Work out the finished part from the listing and answer in its coordinate system (mm). Give positions to 0.01 mm unless a question says otherwise; leave off trailing zeros. Order: outer loops, then holes, each group sorted by start corner. A loop starts at its lowest first (then second) coordinate and runs counter-clockwise, first axis right, second up. Notation, with made-up numbers: (82.25, 85) -> (104.25, 85) arc R12 cw to (104.25, 105) -> close; hole circle Ø6 at (-25.75, -5). An arc over 180 degrees is marked (long way). Use a Markdown table: item, result. Add a question column.
```python
from build123d import *

# Parameters (mm, degrees)
F0_R     = 2.25
F1_DEPTH = 15


with BuildPart() as f1:
    # F0 (on Top) → F1 (new body)
    with BuildSketch(Plane.XY):
        with BuildLine():
            ThreePointArc((20, 0), (18.535534, 3.535534), (15, 5))
            Line((15, 5), (-15, 5))
            ThreePointArc((-15, 5), (-18.535534, 3.535534), (-20, 0))
            ThreePointArc((-20, 0), (-18.535534, -3.535534), (-15, -5))
            Line((-15, -5), (15, -5))
            ThreePointArc((15, -5), (18.535534, -3.535534), (20, 0))
        make_face()
        with Locations((-15, 0)):
            Circle(F0_R, mode=Mode.SUBTRACT)
        with Locations((15, 0)):
            Circle(F0_R, mode=Mode.SUBTRACT)
    extrude(amount=F1_DEPTH)


solid = f1.part
```
1) The part is cut by section C-C, the plane y = 0.5. Determine the outline of the cut face in (x, z).
2) Determine the mould class of faces 1 (the flat face through (0, 0, 0)), 2 (the cylindrical face through (-12.854, 0.676, 7.395)) for opening direction X: released by +X, released by -X, zero draft, split by the parting line, or undercut.
3) The part is cut by section B-B, the plane z = 13.5. Determine the outline of the cut face in (x, y), then the cut area to 3 significant figures.
4) The part is cut by section A-A, the plane x = -16. Determine the outline of the cut face in (y, z), then the cut area to 3 significant figures.
5) Straight lines are drawn through the part: line 1 (Y direction, x = 15, z = 7.5); line 2 (X direction, y = -0.75, z = 5.5); line 3 (X direction, y = -2, z = 8.25). For each, find the intervals that lie inside material, in ascending order.
6) A flat-ended cylindrical pin translates along its axis: pin 1 (1 mm diameter, centred on y = -1.5, z = 5, fed in from +X). Find the tip coordinate at first contact, or state that the pin passes through.
7) The part is cut by section D-D, the plane y = 4. Determine the outline of the cut face in (x, z), then the cut area to 3 significant figures.
A:
| question | item | result |
|---|---|---|
| 1 | outline | (-19.97, 0) -> (-17.19, 0) -> (-17.19, 15) -> (-19.97, 15) -> close; (-12.81, 0) -> (12.81, 0) -> (12.81, 15) -> (-12.81, 15) -> close; (17.19, 0) -> (19.97, 0) -> (19.97, 15) -> (17.19, 15) -> close |
| 2 | face 1 | zero draft |
| 2 | face 2 | undercut |
| 3 | outline | (-15, -5) -> (15, -5) arc R5 ccw to (15, 5) -> (-15, 5) arc R5 ccw to start; hole circle Ø4.5 at (-15, 0); hole circle Ø4.5 at (15, 0) |
| 3 | area | 347 mm^2 |
| 4 | outline | (-4.9, 0) -> (-2.02, 0) -> (-2.02, 15) -> (-4.9, 15) -> close; (2.02, 0) -> (4.9, 0) -> (4.9, 15) -> (2.02, 15) -> close |
| 4 | area | 86.5 mm^2 |
| 5 | line 1 | -5 to -2.25, 2.25 to 5 |
| 5 | line 2 | -19.94 to -17.12, -12.88 to 12.88, 17.12 to 19.94 |
| 5 | line 3 | -19.58 to -16.03, -13.97 to 13.97, 16.03 to 19.58 |
| 6 | pin 1 | x = 19.9 |
| 7 | outline | (-18, 0) -> (18, 0) -> (18, 15) -> (-18, 15) -> close |
| 7 | area | 540 mm^2 |
